Check sheet for the modelled part. Datum: model origin and axes. Units: mm. Round coordinates to 2 decimals unless told otherwise and drop trailing zeros. Order: outer loops, then holes, each group sorted by start corner. A loop starts at its lowest first (then second) coordinate and runs counter-clockwise, first axis right, second up.
```python
from build123d import *

# Parameters (mm, degrees)
F0_R     = 9.5
F1_DEPTH = 150
F3_D     = 6.8
F3_DEPTH = 18.25
F3_TIP   = 2.0429261047
F4_R     = 1
F5_R     = 5


with BuildPart() as f1:
    # F0 (on Front) → F1 (new body)
    with BuildSketch(Plane.XZ):
        Circle(F0_R)
    extrude(amount=F1_DEPTH)

    # F3
    with Locations(Plane.XZ.offset(150)):
        with Locations((0, 0)):
            Hole(F3_D / 2, depth=F3_DEPTH)
            with Locations((0, 0, -(F3_DEPTH + F3_TIP / 2))):  # 118° drill point
                Cone(0, F3_D / 2, F3_TIP, mode=Mode.SUBTRACT)

    # F4
    f4_edges = [f1.edges().sort_by_distance(p)[0] for p in [
        (-9.5, -150, 0),
    ]]
    fillet(f4_edges, radius=F4_R)

    # F5
    f5_edges = [f1.edges().sort_by_distance(p)[0] for p in [
        (9.5, -74.5, 0),
        (-9.5, -149, 0),
        (-9.5, 0, 0),
    ]]
    fillet(f5_edges, radius=F5_R)


solid = f1.part
```
Item 1: Go/stop test with flat-tipped pins: P1, Ø6, axis at x = 4.5, y = -101.5, coming from the -Z side; P2, Ø8, axis at x = 4.5, y = -28, coming from the +Z side; P3, Ø4, axis at x = 0, z = 0, coming from the -Y side. Record where each tip stops, or that it passes through.
Answer:
P1: stops at z = -9.38
P2: stops at z = 9.49
P3: stops at y = -130.91
Item 2: Release check for a two-part mould opening along Z. For faces 1 (the flat face through (4, -150, 0)), 2 (the cylindrical face through (0.74, -140.75, -3.32)), 3 (the conical face through (-0.128, -130.062, -0.576)), 4 (the cylindrical face through (4.38, -75.99, -8.43)) record: released by +Z, released by -Z, zero draft, split by the parting line, or undercut.
Answer:
face 1: zero draft
face 2: undercut
face 3: undercut
face 4: split by the parting line
Item 3: Scan lines: line 1 along Z through (x, y) = (0, -140); line 2 along X through (y, z) = (-89.5, 0.5); line 3 along Z through (x, y) = (0, -39). Record each from-to range of solid material in increasing order.
Answer:
line 1: z = -9.5 to -3.4, 3.4 to 9.5
line 2: x = -9.49 to 9.49
line 3: z = -9.5 to 9.5
Item 4: Sectioned sample at A-A (y = -36). Record the cut outline in (x, z).
Answer:
outline: circle Ø19 at (0, 0)
